from build123d import *

# Parameters (mm, degrees)
SKETCH2_R           = 10
SKETCH2_R_2         = 2
BOSS_EXTRUDE1_DEPTH = 6.35


with BuildPart() as part:
    # Sketch2 → Boss-Extrude1 (new body)
    with BuildSketch(Plane.XY):
        with BuildLine():
            Line((0, 46.5), (500, 46.5))
            ThreePointArc((500, 46.5), (546.5, 0), (500, -46.5))
            Line((500, -46.5), (0, -46.5))
            ThreePointArc((0, -46.5), (-46.5, 0), (0, 46.5))
        make_face()
        Circle(SKETCH2_R, mode=Mode.SUBTRACT)
        with Locations((0, 13.75)):
            Circle(SKETCH2_R_2, mode=Mode.SUBTRACT)
        with Locations((11.907849302, 6.875)):
            Circle(SKETCH2_R_2, mode=Mode.SUBTRACT)
        with Locations((11.907849302, -6.875)):
            Circle(SKETCH2_R_2, mode=Mode.SUBTRACT)
        with Locations((0, -13.75)):
            Circle(SKETCH2_R_2, mode=Mode.SUBTRACT)
        with Locations((-11.907849302, -6.875)):
            Circle(SKETCH2_R_2, mode=Mode.SUBTRACT)
        with Locations((-11.907849302, 6.875)):
            Circle(SKETCH2_R_2, mode=Mode.SUBTRACT)
    extrude(amount=BOSS_EXTRUDE1_DEPTH)


solid = part.part
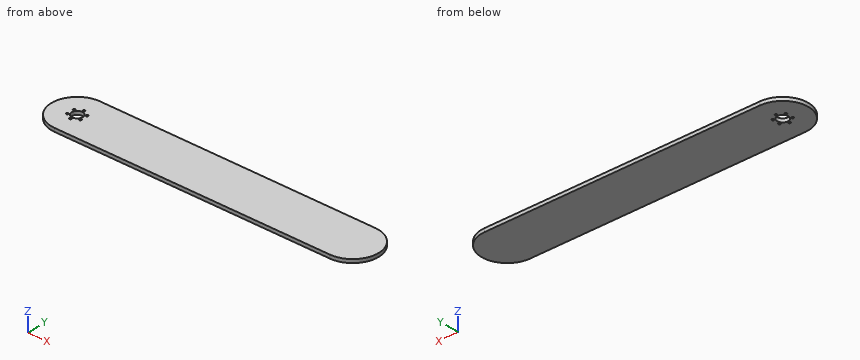
For this review, take the finished solid that the model builds, in its own axes (mm). Give positions to 0.01 mm unless a question says otherwise; leave off trailing zeros. Loops run counter-clockwise (first coordinate to the right, second up) from the corner with the lowest first, then second, coordinate; pieces in that order, holes last. Notation, with made-up numbers: M 14,26 L 45,26 A35 ccw 45,63 Z; hole C 36.5,7.5 d10. An arc over 180 degrees is marked long. Answer as a JSON object with one key per item and string values. Group by question number.
Q1. Add section C-C on y = 25.5. Give the boundary of the cut face in (x, z), and give its area (3 significant figures).
Q2. Insertion check: P1, Ø3, axis at y = -31.5, z = 3, coming from the +X side. The pin has a flat end and moves straight along its axis. Give the tip position at first contact, or say it passes through.
Q3. Add section B-B on z = 1.75. Give the boundary of the cut face in (x, y) (3 decimals).
Q4. For probe 1 along Y at (x, z) = (0, 2); probe 2 along Y at (x, z) = (-5, 1.25); probe 3 along X at (y, z) = (-14, 4.25), list the stretches that pass through material, from the lowest coordinate up. Write a range as [from, to].
Q5. Add section A-A on y = 0. Give the boundary of the cut face in (x, z), and give its area (3 significant figures).
Q6. Add section D-D on y = -28. Give the boundary of the cut face in (x, z).
Checked values:
{
 "1": {"outline": "M -38.88,0 L 538.88,0 L 538.88,6.35 L -38.88,6.35 Z", "area": "3,670 mm²"},
 "2": {"P1": "x = 535.53"},
 "3": {"outline": "M 0,-46.5 L 500,-46.5 A46.5 ccw 500,46.5 L 0,46.5 A46.5 ccw Z; hole C -11.908,-6.875 d4; hole C -11.908,6.875 d4; hole C 0,0 d20; hole C 0,-13.75 d4; hole C 0,13.75 d4; hole C 11.908,-6.875 d4; hole C 11.908,6.875 d4"},
 "4": {"probe 1": "[-46.5, -15.75], [-11.75, -10], [10, 11.75], [15.75, 46.5]", "probe 2": "[-46.23, -8.66], [8.66, 46.23]", "probe 3": "[-44.34, -1.98], [1.98, 544.34]"},
 "5": {"outline": "M -46.5,0 L -10,0 L -10,6.35 L -46.5,6.35 Z; M 10,0 L 546.5,0 L 546.5,6.35 L 10,6.35 Z", "area": "3,640 mm²"},
 "6": {"outline": "M -37.12,0 L 537.12,0 L 537.12,6.35 L -37.12,6.35 Z"}
}
